CAD build for the part. Positions are in the model's coordinates, mm. A direction names the side the tool comes from. Coordinates: 2 decimals unless noted, no trailing zeros. Loops run counter-clockwise (first coordinate to the right, second up) from the corner with the lowest first, then second, coordinate; pieces in that order, holes last. Notation, with made-up numbers: (26, 42) -> (79, 42) arc R17 cw to (79, 50) -> close; hole circle Ø9 at (54.25, 47). An arc over 180 degrees is marked (long way). Answer as a JSON object with one key per item and string values. Group by question number.
from build123d import *

# Parameters (mm, degrees)
SKETCH2_R           = 2.5
SKETCH2_R_2         = 250
BOSS_EXTRUDE1_DEPTH = 20
CUT_EXTRUDE4_DEPTH  = 21
CUT_EXTRUDE5_DEPTH  = 21


with BuildPart() as part:
    # Sketch2 → Boss-Extrude1 (new body)
    with BuildSketch(Plane(origin=(0, 0, 0), x_dir=(1, 0, 0), z_dir=(0, 1, 0))):
        with BuildLine():
            Line((-34.517430478, 903.068960265), (-295.040344804, 95.1377682))
            ThreePointArc((-295.040344804, 95.1377682), (-310, 0), (-295.040344804, -95.1377682))
            Line((-295.040344804, -95.1377682), (-34.517430478, -903.068960265))
            ThreePointArc((-34.517430478, -903.068960265), (-30.886866626, -908.083613135), (-25, -910))
            Line((-25, -910), (25, -910))
            ThreePointArc((25, -910), (30.886866626, -908.083613135), (34.517430478, -903.068960265))
            Line((34.517430478, -903.068960265), (295.040344804, -95.1377682))
            ThreePointArc((295.040344804, -95.1377682), (310, 0), (295.040344804, 95.1377682))
            Line((295.040344804, 95.1377682), (34.517430478, 903.068960265))
            ThreePointArc((34.517430478, 903.068960265), (30.886866626, 908.083613135), (25, 910))
            Line((25, 910), (-25, 910))
            ThreePointArc((-25, 910), (-30.886866626, 908.083613135), (-34.517430478, 903.068960265))
        make_face()
        with Locations((-48.373467006, -762.345774842)):
            Circle(SKETCH2_R, mode=Mode.SUBTRACT)
        with Locations((-94.407870974, -619.584317679)):
            Circle(SKETCH2_R, mode=Mode.SUBTRACT)
        with Locations((-140.442274942, -476.822860516)):
            Circle(SKETCH2_R, mode=Mode.SUBTRACT)
        with BuildLine():
            ThreePointArc((-181.680791071, -251.181388952), (0, -310), (181.680791071, -251.181388952))
            Line((181.680791071, -251.181388952), (9.517430478, -785.092770658))
            ThreePointArc((9.517430478, -785.092770658), (0, -792.023810393), (-9.517430478, -785.092770658))
            Line((-9.517430478, -785.092770658), (-181.680791071, -251.181388952))
        make_face(mode=Mode.SUBTRACT)
        with Locations((-186.476678909, -334.061403353)):
            Circle(SKETCH2_R, mode=Mode.SUBTRACT)
        with Locations((48.373467006, -762.345774842)):
            Circle(SKETCH2_R, mode=Mode.SUBTRACT)
        with Locations((94.407870974, -619.584317679)):
            Circle(SKETCH2_R, mode=Mode.SUBTRACT)
        with Locations((140.442274942, -476.822860516)):
            Circle(SKETCH2_R, mode=Mode.SUBTRACT)
        with Locations((186.476678909, -334.061403353)):
            Circle(SKETCH2_R, mode=Mode.SUBTRACT)
        with Locations((-186.476678909, 334.061403353)):
            Circle(SKETCH2_R, mode=Mode.SUBTRACT)
        with Locations((-140.442274942, 476.822860516)):
            Circle(SKETCH2_R, mode=Mode.SUBTRACT)
        with Locations((-94.407870974, 619.584317679)):
            Circle(SKETCH2_R, mode=Mode.SUBTRACT)
        with BuildLine():
            ThreePointArc((181.680791071, 251.181388952), (0, 310), (-181.680791071, 251.181388952))
            Line((-181.680791071, 251.181388952), (-9.517430478, 785.092770658))
            ThreePointArc((-9.517430478, 785.092770658), (0, 792.023810393), (9.517430478, 785.092770658))
            Line((9.517430478, 785.092770658), (181.680791071, 251.181388952))
        make_face(mode=Mode.SUBTRACT)
        with Locations((-48.373467006, 762.345774842)):
            Circle(SKETCH2_R, mode=Mode.SUBTRACT)
        Circle(SKETCH2_R_2, mode=Mode.SUBTRACT)
        with Locations((186.476678909, 334.061403353)):
            Circle(SKETCH2_R, mode=Mode.SUBTRACT)
        with Locations((140.442274942, 476.822860516)):
            Circle(SKETCH2_R, mode=Mode.SUBTRACT)
        with Locations((94.407870974, 619.584317679)):
            Circle(SKETCH2_R, mode=Mode.SUBTRACT)
        with Locations((48.373467006, 762.345774842)):
            Circle(SKETCH2_R, mode=Mode.SUBTRACT)
    extrude(amount=BOSS_EXTRUDE1_DEPTH)

    # Sketch3 → Cut-Extrude4 (cut, through all)
    with BuildSketch(Plane(origin=(0, 20, 0), x_dir=(1, 0, 0), z_dir=(0, 1, 0))):
        Polygon((-49.523523643, -856.532206403), (-40.006093165, -853.463246139), (-248.695391152, -206.277973666), (-258.21282163, -209.34693393), align=None)
        Polygon((-49.523523643, 856.532206403), (-40.006093165, 853.463246139), (-248.695391152, 206.277973666), (-258.21282163, 209.34693393), align=None)
        Polygon((49.523523643, 856.532206403), (40.006093165, 853.463246139), (248.695391152, 206.277973666), (258.21282163, 209.34693393), align=None)
        Polygon((49.523523643, -856.532206403), (40.006093165, -853.463246139), (248.695391152, -206.277973666), (258.21282163, -209.34693393), align=None)
    extrude(amount=-CUT_EXTRUDE4_DEPTH, mode=Mode.SUBTRACT)

    # Sketch4 → Cut-Extrude5 (cut, through all)
    with BuildSketch(Plane(origin=(0, 20, 0), x_dir=(1, 0, 0), z_dir=(0, 1, 0))):
        Polygon((-255, -100), (-255, 100), (-275, 100), (-275, 30), (-295, 30), (-295, -30), (-275, -30), (-275, -100), align=None)
        Polygon((255, -100), (275, -100), (275, -30), (295, -30), (295, 30), (275, 30), (275, 100), (255, 100), align=None)
    extrude(amount=-CUT_EXTRUDE5_DEPTH, mode=Mode.SUBTRACT)


solid = part.part
Item 1: Band-saw the part on C-C, the plane y = 13. Count the separate pieces of the cut face and the enclosed holes in it, and give its area (3 significant figures).
Item 2: Pull direction X, two halves, no side cores. Call faces 1 (the flat face through (-162, 0, 198)), 2 (the flat face through (-276.9, 9.9, 151.4)), 3 (the flat face through (96.804, 9.86, 514.4)), 4 (the flat face through (276.37, 9.86, 153.04)): +X half, -X half, draft (parallel to the pull), parting line (faces both ways), or undercut.
Item 3: 3-axis set-ups, long thin cutter, end or side, ignore diameter. For faces 5 (the flat face through (-162, 20, 198)), 6 (the flat face through (-96.804, 9.86, -514.4)): which of +Z, -Z, +X, -X, +Y, -Y reach the whole face in a straight line?
Item 4: Band-saw the part on B-B, the plane x = 229.5. List the corners of the cut face in (y, z).
Item 5: Band-saw the part on A-A, the plane z = -117.5. List the corners of the cut face in (x, y), and give its area (3 significant figures).
Item 6: Drill centre lines: L1, parallel to X at y = 19, z = 49; L2, parallel to X at y = 15.5, z = 57; L3, parallel to X at y = 9, z = -506.5. Where is each one in solid material? Low to high.
Item 7: Flat gauge pins, fed straight in: P1, Ø4, axis at x = -186.48, z = -334.06, coming from the -Y side; P2, Ø8, axis at y = 5.5, z = 322.5, coming from the +X side; P3, Ø1, axis at y = 9.5, z = 29, coming from the +X side; P4, Ø2, axis at y = 10, z = 290, coming from the -X side. Where does each tip first touch, or does it go through?
Reply:
{
 "1": {"separate pieces": "1", "enclosed holes": "21", "area": "240,000 mm²"},
 "2": {"face 1": "draft", "face 2": "-X half", "face 3": "undercut", "face 4": "+X half"},
 "3": {"face 5": "+Z, -Z, +X, -X, +Y", "face 6": "+Y, -Y"},
 "4": {"outline": "(0, -265.81) -> (20, -265.81) -> (20, -99.15) -> (0, -99.15) -> close; (0, 99.15) -> (20, 99.15) -> (20, 265.81) -> (0, 265.81) -> close"},
 "5": {"outline": "(-287.83, 0) -> (-220.67, 0) -> (-220.67, 20) -> (-287.83, 20) -> close; (220.67, 0) -> (287.83, 0) -> (287.83, 20) -> (220.67, 20) -> close", "area": "2,690 mm²"},
 "6": {"L1": "-306.1 to -275, -255 to -245.15, 245.15 to 255, 275 to 306.1", "L2": "-304.71 to -275, -255 to -243.42, 243.42 to 255, 275 to 304.71", "L3": "-151.89 to -99.35, 99.35 to 151.89"},
 "7": {"P1": "through", "P2": "x = 212.51", "P3": "x = 308.69", "P4": "x = -222.02"}
}
